```python
from build123d import *

# Parameters (mm, degrees)
F0_R     = 5
F1_DEPTH = 20
F2_SIZE  = 1
F3_SIZE  = 1


with BuildPart() as f1:
    # F0 (on Front) → F1 (new body)
    with BuildSketch(Plane.XZ):
        Circle(F0_R)
    extrude(amount=F1_DEPTH)

    # F2
    f2_edges = [f1.edges().sort_by_distance(p)[0] for p in [
        (-5, 0, 0),
    ]]
    chamfer(f2_edges, length=F2_SIZE)

    # F3
    f3_edges = [f1.edges().sort_by_distance(p)[0] for p in [
        (-5, -20, 0),
    ]]
    chamfer(f3_edges, length=F3_SIZE)


solid = f1.part
```
The listing builds one solid part. Answer for the finished solid, in the listing's coordinates (mm). Round coordinates to 2 decimals unless told otherwise and drop trailing zeros. Loops run counter-clockwise (first coordinate to the right, second up) from the corner with the lowest first, then second, coordinate; pieces in that order, holes last. Notation, with made-up numbers: (86.25, -22.5) - (91.25, -22.5) arc R24 cw to (91.25, 1.5) - close; hole circle Ø8 at (16.25, -3.5). An arc over 180 degrees is marked (long way). Return JSON: item names as keys, results as strings. Group by question number.
1. Each of these flat-tipped pins is pushed along its axis until it touches: P1, Ø5, axis at x = -3.5, y = -8, coming from the +Z side; P2, Ø1, axis at x = -1, y = -11.5, coming from the +Z side; P3, Ø6, axis at y = -8, z = -3.5, coming from the -X side. Where does it stop, or does it pass through?
2. The part is cut by section A-A on y = -11.5. Determine the outline of the cut face in (x, z), then the cut area to 3 significant figures.
3. Consider probe 1 along X at (y, z) = (-8, 2); probe 2 along X at (y, z) = (-8.75, -2.25); probe 3 along Y at (x, z) = (-3.75, 1.75). Determine where each line is inside the solid, lowest interval first.
Resolved:
{
 "1": {"P1": "stops at z = 4.9", "P2": "stops at z = 4.97", "P3": "stops at x = -4.97"},
 "2": {"outline": "circle Ø10 at (0, 0)", "area": "78.5 mm²"},
 "3": {"probe 1": "x = -4.58 to 4.58", "probe 2": "x = -4.47 to 4.47", "probe 3": "y = -19.86 to -0.14"}
}
